```python
from build123d import *

# Parameters (mm, degrees)
SKETCH1_W           = 172.688303012
SKETCH1_H           = 79
SKETCH1_R           = 2.5
BOSS_EXTRUDE1_DEPTH = 10
CUT_EXTRUDE1_REACH  = 81
SKETCH2_W           = 3
SKETCH2_H           = 6.5


with BuildPart() as part:
    # Sketch1 → Boss-Extrude1 (new body)
    with BuildSketch(Plane.XY):
        Rectangle(SKETCH1_W, SKETCH1_H)
        with Locations((3.337204705, -8.386778216)):
            Circle(SKETCH1_R, mode=Mode.SUBTRACT)
    extrude(amount=BOSS_EXTRUDE1_DEPTH)

    # Sketch2 → Cut-Extrude1 (cut, up to next)
    with BuildSketch(Plane(origin=(0, 39.5, 0), x_dir=(1, 0, 0), z_dir=(0, 1, 0)), mode=Mode.PRIVATE) as cut_extrude1_sk1:
        with Locations((84.844151506, -3.25)):
            Rectangle(SKETCH2_W, SKETCH2_H)
    cut_extrude1_tool1 = extrude(cut_extrude1_sk1.sketch, amount=-CUT_EXTRUDE1_REACH, mode=Mode.PRIVATE) & part.part
    add(cut_extrude1_tool1.solids().sort_by_distance((84.844152, 39.5, 3.25))[0], mode=Mode.SUBTRACT)
    # Sketch2 → Cut-Extrude1 (cut, up to next)
    with BuildSketch(Plane(origin=(0, 39.5, 0), x_dir=(1, 0, 0), z_dir=(0, 1, 0)), mode=Mode.PRIVATE) as cut_extrude1_sk2:
        with Locations((50.906490903, -3.25)):
            Rectangle(SKETCH2_W, SKETCH2_H)
    cut_extrude1_tool2 = extrude(cut_extrude1_sk2.sketch, amount=-CUT_EXTRUDE1_REACH, mode=Mode.PRIVATE) & part.part
    add(cut_extrude1_tool2.solids().sort_by_distance((50.906491, 39.5, 3.25))[0], mode=Mode.SUBTRACT)
    # Sketch2 → Cut-Extrude1 (cut, up to next)
    with BuildSketch(Plane(origin=(0, 39.5, 0), x_dir=(1, 0, 0), z_dir=(0, 1, 0)), mode=Mode.PRIVATE) as cut_extrude1_sk3:
        with Locations((16.968830301, -3.25)):
            Rectangle(SKETCH2_W, SKETCH2_H)
    cut_extrude1_tool3 = extrude(cut_extrude1_sk3.sketch, amount=-CUT_EXTRUDE1_REACH, mode=Mode.PRIVATE) & part.part
    add(cut_extrude1_tool3.solids().sort_by_distance((16.96883, 39.5, 3.25))[0], mode=Mode.SUBTRACT)
    # Sketch2 → Cut-Extrude1 (cut, up to next)
    with BuildSketch(Plane(origin=(0, 39.5, 0), x_dir=(1, 0, 0), z_dir=(0, 1, 0)), mode=Mode.PRIVATE) as cut_extrude1_sk4:
        with Locations((-16.968830301, -3.25)):
            Rectangle(SKETCH2_W, SKETCH2_H)
    cut_extrude1_tool4 = extrude(cut_extrude1_sk4.sketch, amount=-CUT_EXTRUDE1_REACH, mode=Mode.PRIVATE) & part.part
    add(cut_extrude1_tool4.solids().sort_by_distance((-16.96883, 39.5, 3.25))[0], mode=Mode.SUBTRACT)
    # Sketch2 → Cut-Extrude1 (cut, up to next)
    with BuildSketch(Plane(origin=(0, 39.5, 0), x_dir=(1, 0, 0), z_dir=(0, 1, 0)), mode=Mode.PRIVATE) as cut_extrude1_sk5:
        with Locations((-50.906490903, -3.25)):
            Rectangle(SKETCH2_W, SKETCH2_H)
    cut_extrude1_tool5 = extrude(cut_extrude1_sk5.sketch, amount=-CUT_EXTRUDE1_REACH, mode=Mode.PRIVATE) & part.part
    add(cut_extrude1_tool5.solids().sort_by_distance((-50.906491, 39.5, 3.25))[0], mode=Mode.SUBTRACT)
    # Sketch2 → Cut-Extrude1 (cut, up to next)
    with BuildSketch(Plane(origin=(0, 39.5, 0), x_dir=(1, 0, 0), z_dir=(0, 1, 0)), mode=Mode.PRIVATE) as cut_extrude1_sk6:
        with Locations((-84.844151506, -3.25)):
            Rectangle(SKETCH2_W, SKETCH2_H)
    cut_extrude1_tool6 = extrude(cut_extrude1_sk6.sketch, amount=-CUT_EXTRUDE1_REACH, mode=Mode.PRIVATE) & part.part
    add(cut_extrude1_tool6.solids().sort_by_distance((-84.844152, 39.5, 3.25))[0], mode=Mode.SUBTRACT)


solid = part.part
```
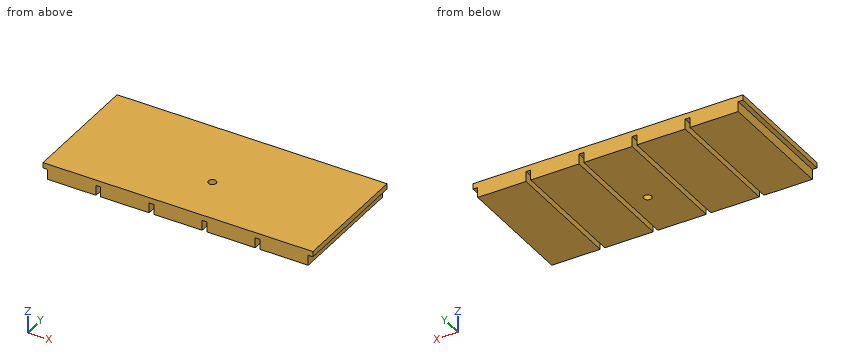
Can you work these out from the model? Positions are in its coordinate system, mm. Give positions to 0.01 mm unless a question says otherwise; leave off trailing zeros. Loops run counter-clockwise (first coordinate to the right, second up) from the corner with the lowest first, then second, coordinate; pieces in that order, holes last. Notation, with made-up numbers: M 37,69.5 L 85,69.5 A17 ccw 85,95.5 Z; hole C -30.75,-26 d9. An arc over 180 degrees is marked long. Use one line per item in the form item = value. Start each with the question number.
(1) Please list where these lines run through material, in increasing order: line 1 (X direction, y = -28.5, z = 2); line 2 (X direction, y = -7, z = 7.5); line 3 (Y direction, x = 5, z = 7).
(2) I'm going to push flat-ended pins straight in: P1, Ø5, axis at y = 11, z = 2.5, coming from the +X side; P2, Ø0.9, axis at x = 84.5, y = 9.5, coming from the -Z side; P3, Ø2, axis at y = -18.5, z = 4, coming from the -X side; P4, Ø4.5, axis at x = 3.34, y = -8.39, coming from the -Z side. Where does each tip first touch, or does it pass through?
(3) I want a section at A-A, the plane y = -30. Write out the boundary of the cut face in (x, z), and give its area (3 significant figures).
Worked out:
q1.line_1 = -83.34 to -52.41, -49.41 to -18.47, -15.47 to 15.47, 18.47 to 49.41, 52.41 to 83.34
q1.line_2 = -86.34 to 1.26, 5.42 to 86.34
q1.line_3 = -39.5 to -10.25, -6.52 to 39.5
q2.P1 = 83.34
q2.P2 = 6.5
q2.P3 = -83.34
q2.P4 = through
q3.outline = M -86.34,6.5 L -83.34,6.5 L -83.34,0 L -52.41,0 L -52.41,6.5 L -49.41,6.5 L -49.41,0 L -18.47,0 L -18.47,6.5 L -15.47,6.5 L -15.47,0 L 15.47,0 L 15.47,6.5 L 18.47,6.5 L 18.47,0 L 49.41,0 L 49.41,6.5 L 52.41,6.5 L 52.41,0 L 83.34,0 L 83.34,6.5 L 86.34,6.5 L 86.34,10 L -86.34,10 Z
q3.area = 1,610 mm²
